Work out the finished part from the listing and answer in its coordinate system (mm). A direction names the side the tool comes from. Give positions to 0.01 mm unless a question says otherwise; leave off trailing zeros. Loops run counter-clockwise (first coordinate to the right, second up) from the corner with the lowest first, then second, coordinate; pieces in that order, holes last. Notation, with made-up numbers: M 12,-33.75 L 25,-33.75 A16 cw 25,-5.75 Z; hole C 42.25,20.5 d5. An arc over 180 degrees is marked long. Use a Markdown table: item, result.
```python
from build123d import *

# Parameters (mm, degrees)
SKETCH1_R           = 2.38125
BOSS_EXTRUDE1_DEPTH = 1.47955
CUT_EXTRUDE1_REACH  = 4.959
CUT_EXTRUDE2_REACH  = 4.959
CUT_EXTRUDE3_DEPTH  = 3.9591


with BuildPart() as part:
    # Sketch1 → Boss-Extrude1 (new body, symmetric)
    with BuildSketch(Plane.XY):
        Polygon((-12.7, 9.525), (12.7, 9.525), (12.7, 12.4841), (22.225, 12.4841), (22.225, 9.525), (31.75, 9.525), (31.75, -9.525), (22.225, -9.525), (22.225, -12.4841), (12.7, -12.4841), (12.7, -9.525), (-12.7, -9.525), (-12.7, -12.4841), (-22.225, -12.4841), (-22.225, -9.525), (-31.75, -9.525), (-31.75, 9.525), (-22.225, 9.525), (-22.225, 12.4841), (-12.7, 12.4841), align=None)
        Circle(SKETCH1_R, mode=Mode.SUBTRACT)
    extrude(amount=BOSS_EXTRUDE1_DEPTH, both=True)

    # Sketch2 → Cut-Extrude1 (cut, up to next)
    with BuildSketch(Plane.XY.offset(1.47955), mode=Mode.PRIVATE) as cut_extrude1_sk1:
        Polygon((-12.7, -3.666174209), (-9.525, -1.833087105), (-9.525, 1.833087105), (-12.7, 3.666174209), (-15.875, 1.833087105), (-15.875, -1.833087105), align=None)
    cut_extrude1_tool1 = extrude(cut_extrude1_sk1.sketch, amount=-CUT_EXTRUDE1_REACH, mode=Mode.PRIVATE) & part.part
    add(cut_extrude1_tool1.solids().sort_by_distance((-12.7, 0, 1.47955))[0], mode=Mode.SUBTRACT)

    # Sketch3 → Cut-Extrude2 (cut, up to next)
    with BuildSketch(Plane.XY.offset(1.47955), mode=Mode.PRIVATE) as cut_extrude2_sk1:
        Polygon((25.4, -3.666174209), (28.575, -1.833087105), (28.575, 1.833087105), (25.4, 3.666174209), (22.225, 1.833087105), (22.225, -1.833087105), align=None)
    cut_extrude2_tool1 = extrude(cut_extrude2_sk1.sketch, amount=-CUT_EXTRUDE2_REACH, mode=Mode.PRIVATE) & part.part
    add(cut_extrude2_tool1.solids().sort_by_distance((25.4, 0, 1.47955))[0], mode=Mode.SUBTRACT)

    # Sketch4 → Cut-Extrude3 (cut, through all)
    with BuildSketch(Plane.XY.offset(1.47955)):
        with BuildLine():
            Line((-12.7, -9.525), (12.7, -9.525))
            ThreePointArc((12.7, -9.525), (0, -7.346024484), (-12.7, -9.525))
        make_face()
    extrude(amount=-CUT_EXTRUDE3_DEPTH, mode=Mode.SUBTRACT)


solid = part.part
```
(1) A cutting plane is placed at D-D (x = -25.5). Write down the section's boundary in (y, z) (3 decimals).
Entries:
| item | result |
|---|---|
| outline | M -9.525,-1.48 L 9.525,-1.48 L 9.525,1.48 L -9.525,1.48 Z |
(2) A cutting plane is placed at B-B (z = -0.8). Count the separate pieces of the cut face and the enclosed holes in it, and give its area (3 significant figures).
Entries:
| item | result |
|---|---|
| separate pieces | 1 |
| enclosed holes | 3 |
| area | 1,200 mm² |
(3) Consider probe 1 along Y at (x, z) = (0, -0.2) (3 decimals); probe 2 along X at (y, z) = (-3, 0.05); probe 3 along X at (y, z) = (-10, 1.25) (3 decimals). Determine where each line is inside the solid, lowest interval first. Write a range as [from, to].
Entries:
| item | result |
|---|---|
| probe 1 | y = [-7.346, -2.381], [2.381, 9.525] |
| probe 2 | x = [-31.75, -13.85], [-11.55, 24.25], [26.55, 31.75] |
| probe 3 | x = [-22.225, -12.7], [12.7, 22.225] |
(4) A cutting plane is placed at A-A (x = 0). Write down the section's boundary in (y, z) (3 decimals).
Entries:
| item | result |
|---|---|
| outline | M -7.346,-1.48 L -2.381,-1.48 L -2.381,1.48 L -7.346,1.48 Z; M 2.381,-1.48 L 9.525,-1.48 L 9.525,1.48 L 2.381,1.48 Z |
(5) Which of the six approach directions +Z, -Z, +X, -X, +Y, -Y give full straight-line access (tool end or side, diameter ignored) to faces 1 (the flat face through (-22.225, -11, 0)), 2 (the flat face through (-11.13, -2.76, 0.02)), 3 (the flat face through (12.7, -11, 0)), 4 (the flat face through (12.7, 11, 0))?
Entries:
| item | result |
|---|---|
| face 1 | +Z, -Z, -X, -Y |
| face 2 | +Z, -Z |
| face 3 | +Z, -Z, -Y |
| face 4 | +Z, -Z, +Y |
(6) A cutting plane is placed at C-C (y = 0). Write down the section's boundary in (x, z) (3 decimals), and give its area (3 significant figures).
Entries:
| item | result |
|---|---|
| outline | M -31.75,-1.48 L -15.875,-1.48 L -15.875,1.48 L -31.75,1.48 Z; M -9.525,-1.48 L -2.381,-1.48 L -2.381,1.48 L -9.525,1.48 Z; M 2.381,-1.48 L 22.225,-1.48 L 22.225,1.48 L 2.381,1.48 Z; M 28.575,-1.48 L 31.75,-1.48 L 31.75,1.48 L 28.575,1.48 Z |
| area | 136 mm² |
(7) The mould has two halves that part along X. Classify faces 5 (the flat face through (26.97, -2.76, 0.02)), 6 (the flat face through (-31.75, 0, 0)), 7 (the flat face through (-27, 9.525, 0)): released by +X, released by -X, zero draft, split by the parting line, or undercut.
Entries:
| item | result |
|---|---|
| face 5 | undercut |
| face 6 | released by -X |
| face 7 | zero draft |
(8) Given P1, Ø0.9, axis at y = -11.5, z = 0.5, coming from the -X side (3 decimals); P2, Ø0.9, axis at y = 10.5, z = 0, coming from the +X side (3 decimals), each flat-ended and moving along its own axis, determine where each tip first touches the part or whether it passes through.
Entries:
| item | result |
|---|---|
| P1 | stops at x = -22.225 |
| P2 | stops at x = 22.225 |
